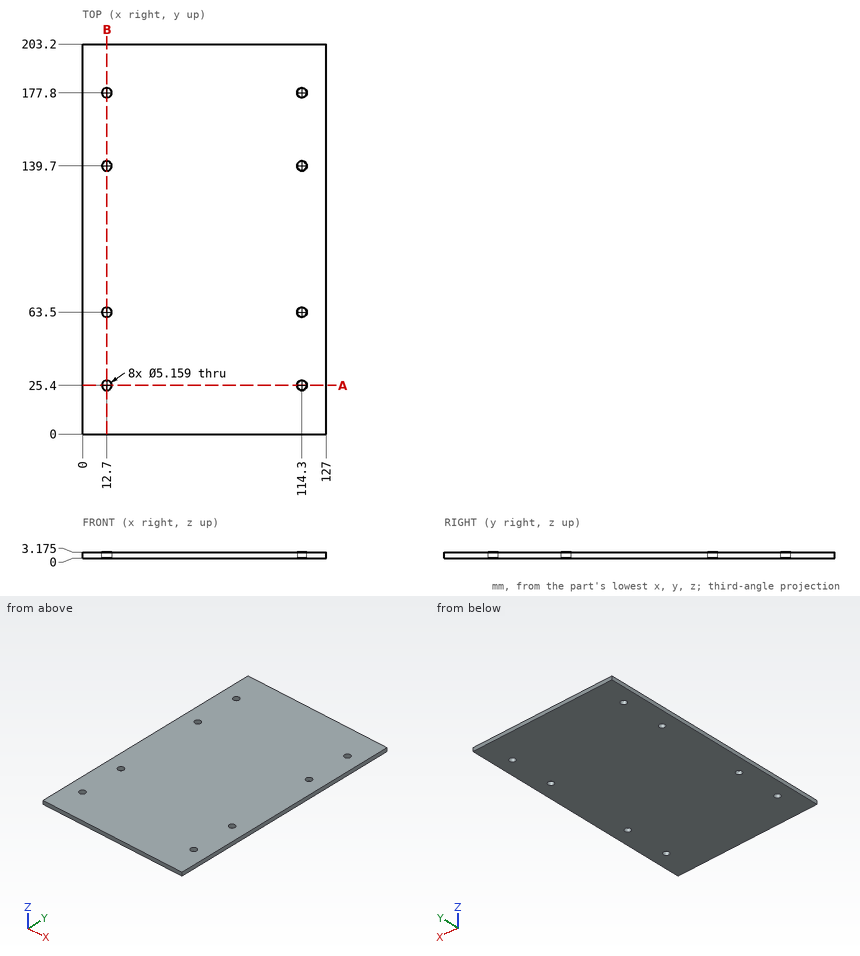
Can you work these out from the drawing? Everything is in mm from the part's minimum corner. Coordinates: 2 decimals unless noted, no trailing zeros. Write each loop counter-clockwise with the first axis right and the second up, starting at its lowest first coordinate (ties: lowest second). Pieces come first, ordered by that corner, then holes. Notation, with made-up numbers: (34, 6) -> (92, 6) arc R32 ccw to (92, 38) -> close; hole circle Ø9 at (-27.5, 78.5). An arc over 180 degrees is marked (long way). Write each question's results on one line, items separated by ' | '. Start each with the question number.
Item 1: Please list where these lines run through material, in increasing order: probe 1 along Y at (x, z) = (12.7, 1.6); probe 2 along X at (y, z) = (139.7, 1.2); probe 3 along Y at (x, z) = (115, 0.65).
Item 2: If we section it at A-A, the plane y = 25.4: Write out the boundary of the cut face in (x, z) (1 decimal).
Item 3: If we section it at B-B, the plane x = 12.7: Write out the boundary of the cut face in (y, z) (1 decimal).
Answer block:
1) probe 1: 0 to 22.82, 27.98 to 60.92, 66.08 to 137.12, 142.28 to 175.22, 180.38 to 203.2 | probe 2: 0 to 10.12, 15.28 to 111.72, 116.88 to 127 | probe 3: 0 to 22.92, 27.88 to 61.02, 65.98 to 137.22, 142.18 to 175.32, 180.28 to 203.2
2) outline: (0, 0) -> (10.1, 0) -> (10.1, 3.2) -> (0, 3.2) -> close; (15.3, 0) -> (111.7, 0) -> (111.7, 3.2) -> (15.3, 3.2) -> close; (116.9, 0) -> (127, 0) -> (127, 3.2) -> (116.9, 3.2) -> close
3) outline: (0, 0) -> (22.8, 0) -> (22.8, 3.2) -> (0, 3.2) -> close; (28, 0) -> (60.9, 0) -> (60.9, 3.2) -> (28, 3.2) -> close; (66.1, 0) -> (137.1, 0) -> (137.1, 3.2) -> (66.1, 3.2) -> close; (142.3, 0) -> (175.2, 0) -> (175.2, 3.2) -> (142.3, 3.2) -> close; (180.4, 0) -> (203.2, 0) -> (203.2, 3.2) -> (180.4, 3.2) -> close
